Verification items for the finished model (mm, model axes). A direction names the side the tool comes from. Round coordinates to 2 decimals unless told otherwise and drop trailing zeros. Write each loop counter-clockwise with the first axis right and the second up, starting at its lowest first coordinate (ties: lowest second). Pieces come first, ordered by that corner, then holes.
from build123d import *


with BuildPart() as f1:
    # F0 (on Front) → F1 (revolve)
    with BuildSketch(Plane.XZ):
        with BuildLine():
            ThreePointArc((75.276984, 16), (75.01005, 15.963715), (74.762488, 15.857493))
            Line((74.762488, 15.857493), (70, 13))
            Line((70, 13), (0, 13))
            Line((0, 13), (0, 0))
            Line((0, 0), (70, 0))
            Line((70, 0), (98, 0))
            Line((98, 0), (115, 0))
            Line((115, 0), (115, 13))
            Line((115, 13), (99, 13))
            ThreePointArc((99, 13), (98.292893, 13.292893), (98, 14))
            Line((98, 14), (98, 16))
            Line((98, 16), (75.276984, 16))
        make_face()
    revolve(axis=Axis((84, 0, 0), (-1, 0, 0)))


solid = f1.part
Q1. Sectioned sample at D-D (x = 97). Enter the section's corners in (y, z), plus the area to 3 significant figures.
Recorded:
outline: circle Ø32 at (0, 0)
area: 804 mm2
Q2. Sectioned sample at A-A (y = 0). Enter the section's corners in (x, z).
Recorded:
outline: (0, -13) - (70, -13) - (74.76, -15.86) arc R1 ccw to (75.28, -16) - (98, -16) - (98, -14) arc R1 cw to (99, -13) - (115, -13) - (115, 13) - (99, 13) arc R1 cw to (98, 14) - (98, 16) - (75.28, 16) arc R1 ccw to (74.76, 15.86) - (70, 13) - (0, 13) - close
Q3. Material ranges on line 1 along Z through (x, y) = (29.5, 5.5); line 2 along Y through (x, z) = (39.5, 11.5); line 3 along Z through (x, y) = (40.5, -10), recorded low to high.
Recorded:
line 1: z = -11.78 to 11.78
line 2: y = -6.06 to 6.06
line 3: z = -8.31 to 8.31
Q4. Tool access check on faces 1 (the flat face through (98, -14.15, 0.07)), 2 (the flat face through (115, 0, 0)), 3 (the cylindrical face through (34.51, -7.91, -10.316)). Record the directions out of +Z, -Z, +X, -X, +Y, -Y that give a thin tool (end or side, any length) a straight path to the whole face; none if there is none.
Recorded:
face 1: +X
face 2: +Z, -Z, +X, +Y, -Y
face 3: -X
Q5. Sectioned sample at C-C (x = 47). Enter the section's corners in (y, z), plus the area to 3 significant figures.
Recorded:
outline: circle Ø26 at (0, 0)
area: 531 mm2
Q6. Depth check by flat-ended pin: P1, Ø2, axis at x = 15, y = -12, coming from the -Z side; P2, Ø12, axis at x = 26.5, y = -7, coming from the -Z side; P3, Ø1.5, axis at x = 16.5, z = 1, coming from the -Y side. Enter the tip coordinate at first touch or a pass-through.
Recorded:
P1: stops at z = -6.93
P2: stops at z = -12.96
P3: stops at y = -13
